The model under review builds one solid part; all positions refer to its coordinate system, in mm. Face numbers are marked on the shaded views. A direction names the side the tool comes from. Coordinates: 2 decimals unless noted, no trailing zeros. Write each loop counter-clockwise with the first axis right and the second up, starting at its lowest first coordinate (ties: lowest second). Pieces come first, ordered by that corner, then holes. Notation, with made-up numbers: M 51.5,0 L 82.5,0 A15 cw 82.5,17 Z; hole C -36,-19.5 d8. An arc over 180 degrees is marked long. Answer as a JSON object with one key per item and string values.
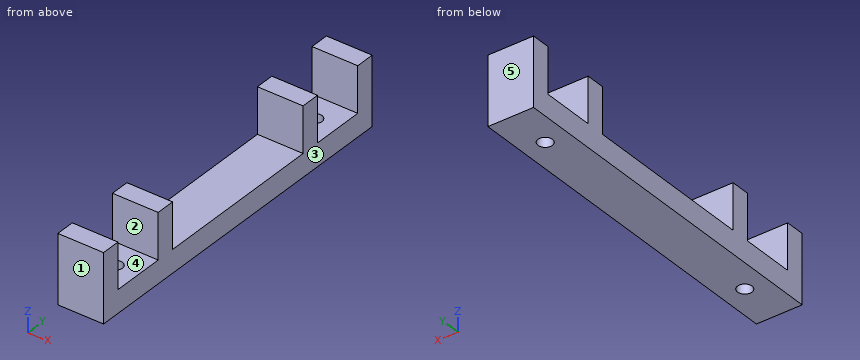
```python
from build123d import *

# Parameters (mm, degrees)
ESQUISSE1_W                    = 6
ESQUISSE1_H                    = 42.7
ESQUISSE1_R                    = 0.95
BOSS_EXTRU_1_DEPTH             = 3
ESQUISSE2_W                    = 6
ESQUISSE2_H                    = 2.5
BOSS_EXTRU_2_DEPTH             = 6
BOSS_EXTRU_2_DIRECTION_2_REACH = 40.932


with BuildPart() as part:
    # Esquisse1 → Boss.-Extru.1 (new body)
    with BuildSketch(Plane.XY):
        with Locations((0, 17.35)):
            Rectangle(ESQUISSE1_W, ESQUISSE1_H)
        Circle(ESQUISSE1_R, mode=Mode.SUBTRACT)
        with Locations((0, 34.7)):
            Circle(ESQUISSE1_R, mode=Mode.SUBTRACT)
    extrude(amount=BOSS_EXTRU_1_DEPTH)

    # Esquisse2 → Boss.-Extru.2 (add)
    with BuildSketch(Plane.XY.offset(3)):
        with Locations((0, 4.75)):
            Rectangle(ESQUISSE2_W, ESQUISSE2_H)
        with Locations((0, 39.45)):
            Rectangle(ESQUISSE2_W, ESQUISSE2_H)
        with Locations((0, 29.95)):
            Rectangle(ESQUISSE2_W, ESQUISSE2_H)
        with Locations((0, -4.75)):
            Rectangle(ESQUISSE2_W, ESQUISSE2_H)
    extrude(amount=BOSS_EXTRU_2_DEPTH)

    # Boss.-Extru.2 direction 2: up to this face of the body (flat: up to its plane)
    boss_extru_2_direction_2_end = Plane(part.part.faces().sort_by_distance((0, 17.35, 0))[0])
    # Esquisse2 → Boss.-Extru.2 direction 2 (add, up to the picked face)
    with BuildSketch(Plane.XY.offset(3), mode=Mode.PRIVATE) as boss_extru_2_direction_2_sk1:
        with Locations((0, 4.75)):
            Rectangle(ESQUISSE2_W, ESQUISSE2_H)
    boss_extru_2_direction_2_tool1 = split(extrude(boss_extru_2_direction_2_sk1.sketch, amount=-BOSS_EXTRU_2_DIRECTION_2_REACH, mode=Mode.PRIVATE), bisect_by=boss_extru_2_direction_2_end, keep=Keep.BOTH, mode=Mode.PRIVATE)
    # Esquisse2 → Boss.-Extru.2 direction 2 (add, up to the picked face)
    with BuildSketch(Plane.XY.offset(3), mode=Mode.PRIVATE) as boss_extru_2_direction_2_sk2:
        with Locations((0, 39.45)):
            Rectangle(ESQUISSE2_W, ESQUISSE2_H)
    boss_extru_2_direction_2_tool2 = split(extrude(boss_extru_2_direction_2_sk2.sketch, amount=-BOSS_EXTRU_2_DIRECTION_2_REACH, mode=Mode.PRIVATE), bisect_by=boss_extru_2_direction_2_end, keep=Keep.BOTH, mode=Mode.PRIVATE)
    # Esquisse2 → Boss.-Extru.2 direction 2 (add, up to the picked face)
    with BuildSketch(Plane.XY.offset(3), mode=Mode.PRIVATE) as boss_extru_2_direction_2_sk3:
        with Locations((0, 29.95)):
            Rectangle(ESQUISSE2_W, ESQUISSE2_H)
    boss_extru_2_direction_2_tool3 = split(extrude(boss_extru_2_direction_2_sk3.sketch, amount=-BOSS_EXTRU_2_DIRECTION_2_REACH, mode=Mode.PRIVATE), bisect_by=boss_extru_2_direction_2_end, keep=Keep.BOTH, mode=Mode.PRIVATE)
    # Esquisse2 → Boss.-Extru.2 direction 2 (add, up to the picked face)
    with BuildSketch(Plane.XY.offset(3), mode=Mode.PRIVATE) as boss_extru_2_direction_2_sk4:
        with Locations((0, -4.75)):
            Rectangle(ESQUISSE2_W, ESQUISSE2_H)
    boss_extru_2_direction_2_tool4 = split(extrude(boss_extru_2_direction_2_sk4.sketch, amount=-BOSS_EXTRU_2_DIRECTION_2_REACH, mode=Mode.PRIVATE), bisect_by=boss_extru_2_direction_2_end, keep=Keep.BOTH, mode=Mode.PRIVATE)
    add(boss_extru_2_direction_2_tool1.solids().sort_by(Axis((0, 4.75, 3), (0, 0, -1)))[0])
    add(boss_extru_2_direction_2_tool2.solids().sort_by(Axis((0, 39.45, 3), (0, 0, -1)))[0])
    add(boss_extru_2_direction_2_tool3.solids().sort_by(Axis((0, 29.95, 3), (0, 0, -1)))[0])
    add(boss_extru_2_direction_2_tool4.solids().sort_by(Axis((0, -4.75, 3), (0, 0, -1)))[0])


solid = part.part
```
(1) For the marked faces 1 and 2, list the 3-axis set-ups (+Z, -Z, +X, -X, +Y, -Y) from which the entire face can be reached by the end or side of a thin tool; tool diameter is ignored.
Results list:
{"face 1": "+Z, -Z, +X, -X, -Y", "face 2": "+Z, +X, -X"}
(2) Draft analysis for pull direction Y (two halves, no side actions). For the marked faces 3, 4 and 5, state which applies: released by +Y, released by -Y, zero draft, split by the parting line, or undercut.
Results list:
{"face 3": "zero draft", "face 4": "undercut", "face 5": "released by +Y"}
(3) Add section D-D on x = 2. Give the boundary of the cut face in (y, z), and give its area (3 significant figures).
Results list:
{"outline": "M -6,0 L 40.7,0 L 40.7,9 L 38.2,9 L 38.2,3 L 31.2,3 L 31.2,9 L 28.7,9 L 28.7,3 L 6,3 L 6,9 L 3.5,9 L 3.5,3 L -3.5,3 L -3.5,9 L -6,9 Z", "area": "200 mm²"}
(4) Add section B-B on z = 5.5. Give the boundary of the cut face in (x, y), and give its area (3 significant figures).
Results list:
{"outline": "M -3,-6 L 3,-6 L 3,-3.5 L -3,-3.5 Z; M -3,3.5 L 3,3.5 L 3,6 L -3,6 Z; M -3,28.7 L 3,28.7 L 3,31.2 L -3,31.2 Z; M -3,38.2 L 3,38.2 L 3,40.7 L -3,40.7 Z", "area": "60.0 mm²"}
(5) Add section C-C on y = 0. Give the boundary of the cut face in (x, z), and give its area (3 significant figures).
Results list:
{"outline": "M -3,0 L -0.95,0 L -0.95,3 L -3,3 Z; M 0.95,0 L 3,0 L 3,3 L 0.95,3 Z", "area": "12.3 mm²"}
(6) Wall thickness on line 1 along Y through (x, z) = (0, 2.3); line 2 along Y through (x, z) = (-1.7, 8.5); line 3 along X through (y, z) = (34.7, 1.75): over which ranges is each line inside the solid? List them lowest first. Write a range as from..to.
Results list:
{"line 1": "-6..-0.95, 0.95..33.75, 35.65..40.7", "line 2": "-6..-3.5, 3.5..6, 28.7..31.2, 38.2..40.7", "line 3": "-3..-0.95, 0.95..3"}
(7) For pin 1 Ø1.5 at (x, y) = (0, 34.7) entering from -Z; pin 2 Ø2 at (x, y) = (-2, 1.5) entering from +Z, all flat-tipped, find the tip position at first contact; note any pin that passes through.
Results list:
{"pin 1": "through", "pin 2": "z = 3"}
(8) Add section A-A on x = 0. Give the boundary of the cut face in (y, z).
Results list:
{"outline": "M -6,0 L -0.95,0 L -0.95,3 L -3.5,3 L -3.5,9 L -6,9 Z; M 0.95,0 L 33.75,0 L 33.75,3 L 31.2,3 L 31.2,9 L 28.7,9 L 28.7,3 L 6,3 L 6,9 L 3.5,9 L 3.5,3 L 0.95,3 Z; M 35.65,0 L 40.7,0 L 40.7,9 L 38.2,9 L 38.2,3 L 35.65,3 Z"}
